from build123d import *

# Parameters (mm, degrees)
BASE_EXTRUDE_DEPTH  = 2
BOSS_EXTRUDE1_DEPTH = 37.16
BOSS_EXTRUDE2_DEPTH = 16.2
FILLET1_R           = 9
SKETCH4_R           = 3.52
CUT_EXTRUDE1_DEPTH  = 64.580171374
FILLET3_R           = 0.5
CUT_EXTRUDE3_START  = -35.16
CUT_EXTRUDE3_DEPTH  = 35.16
BOSS_EXTRUDE3_REACH = 89.266


# Read off the part's stored shape, not the designer's step: Cut-Extrude3
with BuildPart() as part:
    # Sketch1 → Base-Extrude (new body)
    with BuildSketch(Plane.XY):
        with BuildLine():
            Line((54.84113201, -24.576058398), (54.628473973, -23.914611391))
            ThreePointArc((54.628473973, -23.914611391), (51.976550593, -21.839785691), (49.067516522, -23.535403595))
            ThreePointArc((49.067516522, -23.535403595), (22.988082213, -49.326306127), (-13.533918495, -52.710240468))
            ThreePointArc((-13.533918495, -52.710240468), (-16.11871633, -53.245518126), (-17.28, -55.61598691))
            Line((-17.28, -55.61598691), (-17.28, -56.111421297))
            ThreePointArc((-17.28, -56.111421297), (-16.648511043, -57.952658773), (-15.019896373, -59.018748826))
            ThreePointArc((-15.019896373, -59.018748826), (25.543504513, -55.284169318), (54.678638299, -26.815229139))
            ThreePointArc((54.678638299, -26.815229139), (54.977241057, -25.711417004), (54.84113201, -24.576058398))
        make_face()
    extrude(amount=BASE_EXTRUDE_DEPTH)

    # Sketch2 → Boss-Extrude1 (add)
    with BuildSketch(Plane.XY.offset(2)):
        with BuildLine():
            Line((-15.28, -55.61598691), (-15.28, -56.111421297))
            ThreePointArc((-15.28, -56.111421297), (-15.069503681, -56.725167122), (-14.526632124, -57.080530473))
            ThreePointArc((-14.526632124, -57.080530473), (24.70463737, -53.468597255), (52.882952312, -25.934597641))
            ThreePointArc((52.882952312, -25.934597641), (52.982486565, -25.566660262), (52.937116882, -25.188207393))
            Line((52.937116882, -25.188207393), (52.724458845, -24.526760386))
            ThreePointArc((52.724458845, -24.526760386), (51.840484385, -23.83515182), (50.870806361, -24.400357788))
            ThreePointArc((50.870806361, -24.400357788), (23.832921691, -51.139106794), (-14.031306165, -54.647404763))
            ThreePointArc((-14.031306165, -54.647404763), (-14.892905443, -54.825830649), (-15.28, -55.61598691))
        make_face()
    extrude(amount=-BOSS_EXTRUDE1_DEPTH)

    # Sketch3 → Boss-Extrude2 (add)
    with BuildSketch(Plane.XY.offset(2)):
        Polygon((31.667200425, -46.643561321), (33.187911486, -49.906602521), (16.872705491, -57.510157828), (15.351994429, -54.247116629), align=None)
    extrude(amount=BOSS_EXTRUDE2_DEPTH)

    # Fillet1
    fillet1_edges = [part.edges().sort_by_distance(p)[0] for p in [
        (16.11234996, -55.878637228, 18.2),
        (32.427555956, -48.275081921, 18.2),
    ]]
    fillet(fillet1_edges, radius=FILLET1_R - 0.0001)  # a hair under: the kernel refuses the full size

    # Sketch4 → Cut-Extrude1 (cut, through all)
    with BuildSketch(Plane(origin=(25.030308488, -53.708380174, 0), x_dir=(0.9064003331019249, 0.4224197393028875, 0), z_dir=(0.42241973930288756, -0.906400333101925, 0))):
        with Locations((0, 9.2)):
            Circle(SKETCH4_R)
    extrude(amount=-CUT_EXTRUDE1_DEPTH, mode=Mode.SUBTRACT)

    # Fillet3
    fillet3_edges = [part.edges().sort_by_distance(p)[0] for p in [
        (54.977241057, -25.711417004, 2),
        (25.543504513, -55.284169318, 0),
        (-16.648511043, -57.952658773, 0),
        (54.734802991, -24.245334894, 2),
        (51.976550593, -21.839785691, 2),
        (22.988082213, -49.326306127, 2),
        (-16.11871633, -53.245518126, 2),
        (-17.28, -55.863704104, 2),
        (-16.648511043, -57.952658773, 2),
        (25.543504513, -55.284169318, 2),
        (16.872705491, -57.510157828, 5.60005),
        (15.351994429, -54.247116629, 5.60005),
        (31.667200425, -46.643561321, 5.60005),
        (29.277920373, -47.757063843, 15.56399032),
        (17.741274481, -53.133614107, 15.56399032),
        (33.187911486, -49.906602521, 5.60005),
        (30.798631434, -51.020105042, 15.56399032),
        (-17.28, -55.863704104, 0),
        (19.261985543, -56.396655306, 15.56399032),
        (-16.11871633, -53.245518126, 0),
        (22.988082213, -49.326306127, 0),
        (51.976550593, -21.839785691, 0),
        (54.734802991, -24.245334894, 0),
        (54.977241057, -25.711417004, 0),
    ]]
    fillet(fillet3_edges, radius=FILLET3_R)

    # Cut-Extrude3 outline → Cut-Extrude3 (cut)
    with BuildSketch(Plane(origin=(0, 0, -35.16), x_dir=(-1, 0, 0), z_dir=(0, 0, -1)).offset(CUT_EXTRUDE3_START)):
        with BuildLine():
            Line((-31.685344985, -46.682494719), (-32.404496034, -48.225601466))
            Line((-32.404496034, -48.225601466), (-16.089290038, -55.829156774))
            Line((-16.089290038, -55.829156774), (-15.370138989, -54.286050026))
            ThreePointArc((-15.370138989, -54.286050026), (-23.832921691, -51.139106794), (-31.685344985, -46.682494719))
        make_face()
    extrude(amount=CUT_EXTRUDE3_DEPTH, mode=Mode.SUBTRACT)

    # Sketch7 → Boss-Extrude3 (add, up to next)
    with BuildSketch(Plane(origin=(8.157602998, 3.801777654, 0), x_dir=(0, 0, 1), z_dir=(-0.9064003331019256, -0.42241973930288634, 0)), mode=Mode.PRIVATE) as boss_extrude3_sk1:
        with BuildLine():
            Line((-25.66, -57.4), (-22.16, -55.697543931))
            Line((-22.16, -55.697543931), (-21.16, -57.4))
            ThreePointArc((-21.16, -57.4), (-20.56, -56.8), (-19.96, -57.4))
            Line((-19.96, -57.4), (-21.16, -57.566686604))
            Line((-21.16, -57.566686604), (-25.66, -57.4))
        make_face()
    boss_extrude3_tool1 = extrude(boss_extrude3_sk1.sketch, amount=BOSS_EXTRUDE3_REACH, mode=Mode.PRIVATE) - part.part
    add(boss_extrude3_tool1.solids().sort_by_distance((32.205788, -47.799227, -22.639326))[0])
    add(boss_extrude3_tool1.solids().sort_by_distance((32.205788, -47.799227, -22.639326))[1])


solid = part.part
Could you check a few things on this model? Use its own coordinates, in mm. A direction names the side the tool comes from. Coordinates: 2 decimals unless noted, no trailing zeros. Loops run counter-clockwise (first coordinate to the right, second up) from the corner with the lowest first, then second, coordinate; pieces in that order, holes last.
1. I need wall thicknesses on L1, parallel to Z at x = 4, y = -58.5; L2, parallel to Y at x = 6, z = -21; L3, parallel to X at y = -28, z = -33. Which ranges of each line are inside material? Lowest first, please.
2. Imagine slicing it at A-A (z = -27.5). Please give me the cut outline in (x, y).
3. We'd pull the mould along Z, two halves only. Please class faces 1 (the face through (15.735, -55.068, -10.925)), 2 (the face through (51.857, -23.836, -17.334)), 3 (the face through (30.109, -49.376, 15.494)), 4 (the face through (24.361, -51.974, -9.84)): released by +Z, released by -Z, zero draft, split by the parting line, or undercut.
4. For P1, Ø4, axis at x = 23.5, z = -10.5, coming from the +Y side; P2, Ø12, axis at y = -29.5, z = -19, coming from the -X side; P3, Ø1, axis at y = -29, z = -18, coming from the -X side; P4, Ø11.5, axis at x = 15, y = -44.5, coming from the -Z side, each with a flat end and sliding along its axis, tell me the tip position at first contact or that it passes through.
5. For faces 5 (the face through (15.735, -55.068, -30.013)), 6 (the face through (26.83, -48.9, 9.74)), 7 (the face through (42.891, -36.655, -17.334)), which set-ups out of +Z, -Z, +X, -X, +Y, -Y let a thin tool reach every point of the face, with its end or its side?
Computed values:
1. L1: z = -35.16 to 2
1. L2: y = -58.59 to -56.1
1. L3: x = 48.98 to 51.82
2. outline: (-15.28, -56.11) arc R1 ccw to (-14.53, -57.08) arc R58.9 ccw to (52.88, -25.93) arc R1 ccw to (52.94, -25.19) - (52.72, -24.53) arc R1 ccw to (50.87, -24.4) arc R56.42 cw to (31.69, -46.68) - (32.4, -48.23) - (16.09, -55.83) - (15.37, -54.29) arc R56.42 cw to (-14.03, -54.65) arc R1 ccw to (-15.28, -55.62) - close
3. face 1: undercut
3. face 2: zero draft
3. face 3: released by +Z
3. face 4: undercut
4. P1: stops at y = -51.44
4. P2: stops at x = 43.85
4. P3: stops at x = 48.09
4. P4: passes through
5. face 5: -Z, +Y
5. face 6: +Z, -X, +Y
5. face 7: -Z, -X, +Y
